from build123d import *

# Parameters (mm, degrees)
F0_W     = 72.952986
F0_H     = 66.589336
F1_DEPTH = 50.8
F2_R     = 5.08
F4_D     = 6.35


with BuildPart() as f1:
    # F0 (on Front) → F1 (new body)
    with BuildSketch(Plane.XZ):
        Rectangle(F0_W, F0_H)
    extrude(amount=F1_DEPTH)

    # F2
    f2_edges = [f1.edges().sort_by_distance(p)[0] for p in [
        (36.476493, -25.4, 33.294668),
        (0, -50.8, 33.294668),
        (-36.476493, -25.4, 33.294668),
        (0, 0, 33.294668),
    ]]
    fillet(f2_edges, radius=F2_R)

    # F4 (through all)
    with Locations(Plane.XY.offset(33.294668)):
        with Locations((-18.866701, -25.4), (19.233299, -25.4)):
            Hole(F4_D / 2)


solid = f1.part
Design review of the part built by this model. Coordinates are the model's own, in mm. Round coordinates to 2 decimals unless told otherwise and drop trailing zeros. Loops run counter-clockwise (first coordinate to the right, second up) from the corner with the lowest first, then second, coordinate; pieces in that order, holes last. Notation, with made-up numbers: (2, -29) - (21, -29) arc R28 cw to (21, 2) - close; hole circle Ø4 at (77.25, -35). An arc over 180 degrees is marked (long way). One line per item, written item: value. Start each with the question number.
1) Insertion check: pin 1 Ø5 at (x, y) = (17.5, -24.5) entering from -Z. The pin has a flat end and moves straight along its axis. Give the tip position at first contact, or say it passes through.
2) Consider section B-B on z = -25.5. Give the number of separate pieces and of enclosed holes in the cut face, then the cut area to 3 significant figures.
3) Consider section A-A on y = -25.4. Give the boundary of the cut face in (x, z).
4) Draft analysis for pull direction X (two halves, no side actions). For faces 1 (the flat face through (-1, -25, -33.295)), 2 (the cylindrical face through (35.028, -25.756, 31.767)), 3 (the cylindrical face through (21.57, -23.25, -0.47)), state which applies: +X half, -X half, draft (parallel to the pull), parting line (faces both ways), or undercut.
5) To check wall thickness, follow L1, parallel to X at y = -25, z = 14; L2, parallel to Y at x = -17.5, z = -8; L3, parallel to Y at x = -19.5, z = 28.5. State the ranges of each line that lie inside material, in increasing order. Write a range as from..to.
Reported:
1. pin 1: stops at z = -33.29
2. separate pieces: 1
2. enclosed holes: 2
2. area: 3,640 mm^2
3. outline: (-36.48, -33.29) - (-22.04, -33.29) - (-22.04, 33.29) - (-31.4, 33.29) arc R5.08 ccw to (-36.48, 28.21) - close; (-15.69, -33.29) - (16.06, -33.29) - (16.06, 33.29) - (-15.69, 33.29) - close; (22.41, -33.29) - (36.48, -33.29) - (36.48, 28.21) arc R5.08 ccw to (31.4, 33.29) - (22.41, 33.29) - close
4. face 1: draft
4. face 2: +X half
4. face 3: undercut
5. L1: x = -36.48..-22.02, -15.72..16.08, 22.38..36.48
5. L2: y = -50.8..-28.27, -22.53..0
5. L3: y = -50.79..-28.51, -22.29..-0.01
